Autodesk Inventor part; units mm, degrees
ref_plane "right_body_XY" through (0, 0, 0) normal (0, 0, -1) x (1, 0, 0)
ref_plane "right_body_YZ" through (0, 0, 0) normal (1, 0, 0) x (0, -1, 0)
ref_plane "right_body_ZX" through (0, 0, 0) normal (0, -1, 0) x (0, 0, -1)
sketch "Sketch_1" plane through (0, 0, 0) normal (0, 0, 1) x (1, 0, 0)
  line L0 (-3.8862, 2.413) -> (-3.8862, -2.413)
  line L1 (-3.8862, -2.413) -> (3.8862, -2.413)
  line L2 (3.8862, -2.413) -> (3.8862, 2.413)
  line L3 (3.8862, 2.413) -> (-3.8862, 2.413)
extrude "Extrusion1" add sketch "Sketch_1" against normal blind 0.0254
sketch "Sketch_2" plane through (0, 0, -1.0414) normal (0, 0, 1) x (1, 0, 0)
  circle A0 centre (-2.54, -0.9906) radius 0.3048
extrude "Extrusion2" add sketch "Sketch_2" along normal blind 1.0414
sketch "Sketch_5" plane through (0, 0, -1.0414) normal (0, 0, 1) x (1, 0, 0)
  circle A0 centre (2.54, -0.9906) radius 0.3048
extrude "Extrusion3" add sketch "Sketch_5" along normal blind 1.0414
sketch "Sketch_6" plane through (0, 0, -1.0414) normal (0, 0, 1) x (1, 0, 0)
  line L0 (3.81, -1.6002) -> (-3.81, -1.6002)
  circle A0 centre (-2.54, -0.9906) radius 0.3048
revolve "Revolution1" add sketch "Sketch_6" angle 90 about axis through (3.81, -1.6002, -1.0414) along (-1, 0, 0)
sketch "Sketch_7" plane through (0, 0, -1.0414) normal (0, 0, 1) x (1, 0, 0)
  line L0 (2.54, -1.6002) -> (-2.54, -1.6002)
  circle A0 centre (2.54, -0.9906) radius 0.3048
revolve "Revolution2" add sketch "Sketch_7" angle 90 about axis through (2.54, -1.6002, -1.0414) along (-1, 0, 0)
sketch "Sketch_9" plane through (0, -1.6002, 0) normal (0, 1, 0) x (1, 0, 0)
  circle A0 centre (-2.54, 1.651) radius 0.3048
extrude "Extrusion4" add sketch "Sketch_9" against normal blind 4.826
sketch "Sketch_10" plane through (0, -1.6002, 0) normal (0, 1, 0) x (1, 0, 0)
  circle A0 centre (2.54, 1.651) radius 0.3048
extrude "Extrusion5" add sketch "Sketch_10" against normal blind 4.826
ref_plane "right_body_XY" through (0, 0, 0) normal (0, 0, -1) x (1, 0, 0)
ref_plane "right_body_YZ" through (0, 0, 0) normal (1, 0, 0) x (0, -1, 0)
ref_plane "right_body_ZX" through (0, 0, 0) normal (0, -1, 0) x (0, 0, -1)
properties part number "AS11CHtrh"
Input: part model. Units: mm. Frame: model coordinates. Give positions to 0.01 mm unless a question says otherwise; leave off trailing zeros. Order: outer loops, then holes, each group sorted by start corner. A loop starts at its lowest first (then second) coordinate and runs counter-clockwise, first axis right, second up. Notation, with made-up numbers: M 26.25,43.5 L 45.25,43.5 A33 ccw 45.25,81.5 Z; hole C -13,26.5 d1. An arc over 180 degrees is marked long. Answer as a JSON object with one key per item and string values.
1. Cut plane C-C, the plane z = -0.8. Output: boundary loops of the cut face in (x, y).
Result sheet:
{"outline": "C -2.54,-0.99 d0.61; C 2.54,-0.99 d0.61"}
2. Ray query, line 1 (X direction, y = -1, z = -1.35); line 2 (Z direction, x = 2.5, y = -3); line 3 (X direction, y = -4.5, z = -1.55). Return the intervals inside material, ascending. Write a range as [from, to].
Result sheet:
{"line 1": "[-2.84, -2.24], [2.24, 2.84]", "line 2": "[-1.95, -1.35]", "line 3": "[-2.83, -2.25], [2.25, 2.83]"}
3. Cut plane D-D, the plane y = -3.75. Output: boundary loops of the cut face in (x, z).
Result sheet:
{"outline": "C -2.54,-1.65 d0.61; C 2.54,-1.65 d0.61"}
4. First-contact query: P1, Ø1.4, axis at x = 2, y = -0.5, coming from the -Z side; P2, Ø2, axis at x = 2, y = -4, coming from the +Z side; P3, Ø1.5, axis at x = 2, y = -0.5, coming from the -Z side. Flat tips, straight axial feed; report the tip coordinate or a pass-through.
Result sheet:
{"P1": "z = -1.75", "P2": "z = -1.35", "P3": "z = -1.79"}
5. Cut plane B-B, the plane y = -1.75. State how many separate pieces and enclosed holes the cut face has, and give its area (3 significant figures).
Result sheet:
{"separate pieces": "3", "enclosed holes": "0", "area": "0.781 mm²"}
